```python
from build123d import *

# Parameters (mm, degrees)
F1_DEPTH = 8
F2_R     = 1.9
F3_DEPTH = 8.001
F5_DEPTH = 3
F6_ANGLE = 90


with BuildPart() as f1:
    # F0 (on Top) → F1 (new body)
    with BuildSketch(Plane.XY):
        with BuildLine():
            ThreePointArc((-0.125, 4.9984372558), (-3.6656130115, 3.4004825025), (-4.99375, -0.2499218628))
            ThreePointArc((-4.99375, -0.2499218628), (0.125, -4.9984372558), (5, 0))
            ThreePointArc((5, 0), (3.4910600109, 3.5794552658), (-0.125, 4.9984372558))
        make_face()
        with BuildLine():
            Line((-8.99125, 79.6251054846), (-4.99375, -0.2499218628))
            ThreePointArc((-4.99375, -0.2499218628), (-3.6656130115, 3.4004825025), (-0.125, 4.9984372558))
            Line((-0.125, 4.9984372558), (-1.825, 72.9771839344))
            ThreePointArc((-1.825, 72.9771839344), (-6.7606755035, 74.8431378764), (-8.99125, 79.6251054846))
        make_face()
        with BuildLine():
            ThreePointArc((-0.125, 4.9984372558), (3.4910600109, 3.5794552658), (5, 0))
            Line((5, 0), (5, 79.9749960925))
            ThreePointArc((5, 79.9749960925), (3.0112373721, 75.0875120772), (-1.825, 72.9771839344))
            Line((-1.825, 72.9771839344), (-0.125, 4.9984372558))
        make_face()
        with BuildLine():
            ThreePointArc((-5, 86.2995514129), (-8.0077721539, 83.567582034), (-8.99125, 79.6251054846))
            ThreePointArc((-8.99125, 79.6251054846), (-6.7606755035, 74.8431378764), (-1.825, 72.9771839344))
            Line((-1.825, 72.9771839344), (-2, 79.9749960925))
            Line((-2, 79.9749960925), (-5, 79.9749960925))
            Line((-5, 79.9749960925), (-5, 86.2995514129))
        make_face()
        with BuildLine():
            Line((-2, 79.9749960925), (5, 79.9749960925))
            ThreePointArc((5, 79.9749960925), (1.7416573868, 85.8910758756), (-5, 86.2995514129))
            Line((-5, 86.2995514129), (-5, 79.9749960925))
            Line((-5, 79.9749960925), (-2, 79.9749960925))
        make_face()
        with BuildLine():
            ThreePointArc((-1.825, 72.9771839344), (3.0112373721, 75.0875120772), (5, 79.9749960925))
            Line((5, 79.9749960925), (-2, 79.9749960925))
            Line((-2, 79.9749960925), (-1.825, 72.9771839344))
        make_face()
        with BuildLine():
            ThreePointArc((-5, 86.2995514129), (1.7416573868, 85.8910758756), (5, 79.9749960925))
            Line((5, 79.9749960925), (5, 114.9749960925))
            ThreePointArc((5, 114.9749960925), (1.8301270189, 108.8512717356), (-5, 107.9039282807))
            Line((-5, 107.9039282807), (-5, 86.2995514129))
        make_face()
        with BuildLine():
            ThreePointArc((-5, 107.9039282807), (1.8301270189, 108.8512717356), (5, 114.9749960925))
            Line((5, 114.9749960925), (-5, 114.9749960925))
            Line((-5, 114.9749960925), (-5, 107.9039282807))
        make_face()
        with BuildLine():
            Line((-5, 114.9749960925), (5, 114.9749960925))
            ThreePointArc((5, 114.9749960925), (-6.8301270189, 121.0987204495), (-5, 107.9039282807))
            Line((-5, 107.9039282807), (-5, 114.9749960925))
        make_face()
    extrude(amount=F1_DEPTH)

    # F2 (on face) → F3 (cut, through all)
    with BuildSketch(Plane.XY.offset(8)):
        with Locations((-2, 79.9749960925)):
            Circle(F2_R)
        with Locations((-2.5, 114.9749960925)):
            Circle(F2_R)
        Circle(F2_R)
    extrude(amount=-F3_DEPTH, mode=Mode.SUBTRACT)

    # F4 (on face) → F5 (cut)
    with BuildSketch(Plane.XY.offset(8)):
        with BuildLine():
            ThreePointArc((-2.99625, -0.1499531177), (0.075, -2.9990623535), (3, 0))
            Line((3, 0), (3, 79.9749960925))
            ThreePointArc((3, 79.9749960925), (0.6726124191, 84.2007673662), (-4.1428571429, 84.4925356071))
            ThreePointArc((-4.1428571429, 84.4925356071), (-6.2912658242, 82.5411289079), (-6.99375, 79.7250742297))
            Line((-6.99375, 79.7250742297), (-2.99625, -0.1499531177))
        make_face()
    extrude(amount=-F5_DEPTH, mode=Mode.SUBTRACT)


with BuildPart() as f1_1:
    # F6: moved
    add(f1.part.rotate(Axis((0, 0, 5), (0, 0, 1)), F6_ANGLE))


solid = f1_1.part
```
Design review of the part built by this model. Coordinates are the model's own, in mm. A direction names the side the tool comes from. Give positions to 0.01 mm unless a question says otherwise; leave off trailing zeros. Write each loop counter-clockwise with the first axis right and the second up, starting at its lowest first coordinate (ties: lowest second). Pieces come first, ordered by that corner, then holes. Notation, with made-up numbers: (-36, -1) -> (14, -1) arc R21 ccw to (14, 22) -> close; hole circle Ø1 at (44, 58.25). An arc over 180 degrees is marked (long way). Answer in a Markdown table with one row per item.
(1) For faces 5 (the flat face through (-42, -1, 5)), 6 (the flat face through (-97, -5, 4)), 7 (the flat face through (-57, 5, 4)), list the 3-axis set-ups (+Z, -Z, +X, -X, +Y, -Y) from which the entire face can be reached by the end or side of a thin tool; tool diameter is ignored.
Results:
| item | result |
|---|---|
| face 5 | +Z |
| face 6 | +Z, -Z, -Y |
| face 7 | +Z, -Z, +X, -X, +Y |
(2) Consider section D-D (x = -14.5). State the section outline as (y, z) points, then the cut area to 3 significant figures.
Results:
| item | result |
|---|---|
| outline | (-5.73, 0) -> (5, 0) -> (5, 8) -> (3, 8) -> (3, 5) -> (-3.73, 5) -> (-3.73, 8) -> (-5.73, 8) -> close |
| area | 65.7 mm2 |
(3) Consider section C-C (x = -90.5). State the section outline as (y, z) points.
Results:
| item | result |
|---|---|
| outline | (-5, 0) -> (5, 0) -> (5, 8) -> (-5, 8) -> close |
(4) Consider section B-B (x = -75.5). State the section outline as (y, z) points, then the cut area to 3 significant figures.
Results:
| item | result |
|---|---|
| outline | (-8.78, 0) -> (5, 0) -> (5, 8) -> (3, 8) -> (3, 5) -> (-6.78, 5) -> (-6.78, 8) -> (-8.78, 8) -> close |
| area | 80.9 mm2 |
(5) Mouldability with a two-part tool opening along Y and no side actions: class faces 1 (the cylindrical face through (-78.12, -2.41, 2.54)), 2 (the flat face through (-40.25, -7.02, 3.94)), 3 (the flat face through (-74, 4, 8)), 4 (the cylindrical face through (-0.571, 1.812, 2.535)) as +Y half, -Y half, draft (parallel to the pull), parting line (faces both ways), or undercut.
Results:
| item | result |
|---|---|
| face 1 | undercut |
| face 2 | -Y half |
| face 3 | draft |
| face 4 | undercut |
(6) To check wall thickness, follow probe 1 along X at (y, z) = (-3, 4.75); probe 2 along Z at (x, y) = (-73, -3.5); probe 3 along X at (y, z) = (-2, 3.4) (3 decimals). State the ranges of each line that lie inside material, in increasing order.
Results:
| item | result |
|---|---|
| probe 1 | -122.46 to -116.81, -113.14 to -81.59, -78.36 to 4 |
| probe 2 | 0 to 5 |
| probe 3 | -122.458 to -116.808, -113.142 to -81.875, -78.075 to 4.583 |
(7) Consider section A-A (z = 2). State the section outline as (x, y) points (3 decimals).
Results:
| item | result |
|---|---|
| outline | (-114.975, 5) arc R7.5 ccw (long way) to (-107.904, -5) -> (-86.3, -5) arc R7 ccw to (-79.625, -8.991) -> (0.25, -4.994) arc R5 ccw to (0, 5) -> close; hole circle Ø3.8 at (-114.975, -2.5); hole circle Ø3.8 at (-79.975, -2); hole circle Ø3.8 at (0, 0) |
(8) Clearance check with flat-ended pins moving along their axes: pin 1 (1.5 mm diameter, centred on x = -57.5, z = 2, fed in from -Y); pin 2 (3.5 mm diameter, centred on x = -57.5, z = 6.5, fed in from -Y); pin 3 (3.5 mm diameter, centred on x = -114.97, y = -2.5, fed in from -Z). State where each tip first meets the part, or that it passes through.
Results:
| item | result |
|---|---|
| pin 1 | y = -7.92 |
| pin 2 | y = -7.97 |
| pin 3 | through |
